```python
from build123d import *

# Parameters (mm, degrees)
ESBO_O1_R                         = 10
RESSALTO_EXTRUS_O1_DEPTH          = 88
ESBO_O1_6_W                       = 24
ESBO_O1_6_H                       = 20
RESSALTO_EXTRUS_O2_DEPTH          = 56
CORTE_EXTRUS_O1_REACH             = 126.957
CORTE_EXTRUS_O1_DIRECTION_2_REACH = 126.957
CORTE_EXTRUS_O2_DEPTH             = 50
CORTE_EXTRUS_O6_REACH             = 126.5
CORTE_EXTRUS_O6_END_RADIUS        = 10
ESBO_O3_R                         = 6
FILETE1_R                         = 3
FILETE2_R                         = 3


with BuildPart() as part:
    # Esboço1 → Ressalto-extrusão1 (new body)
    with BuildSketch(Plane.XY):
        with BuildLine():
            Line((-60, 25), (-48, 25))
            Line((-48, 25), (-48, 35))
            Line((-48, 35), (-42, 35))
            Line((-42, 35), (-42, 50))
            Line((-42, 50), (-18, 50))
            Line((-18, 50), (-18, 35))
            Line((-18, 35), (-12, 35))
            Line((-12, 35), (-12, 25))
            Line((-12, 25), (0, 25))
            ThreePointArc((0, 25), (12.5, 12.5), (0, 0))
            Line((0, 0), (-60, 0))
            ThreePointArc((-60, 0), (-72.5, 12.5), (-60, 25))
        make_face()
        with Locations((-30, 25)):
            Circle(ESBO_O1_R, mode=Mode.SUBTRACT)
    extrude(amount=-RESSALTO_EXTRUS_O1_DEPTH)

    # Esboço1<6> → Ressalto-extrusão2 (add)
    with BuildSketch(Plane.XY):
        with Locations((-30, 60)):
            Rectangle(ESBO_O1_6_W, ESBO_O1_6_H)
    extrude(amount=-RESSALTO_EXTRUS_O2_DEPTH)

    # Esboço2 → Corte-extrusão1 (cut, up to next)
    with BuildSketch(Plane.ZY.offset(42), mode=Mode.PRIVATE) as corte_extrus_o1_sk1:
        Polygon((-40.414518843, 70), (0, 0), (0, 70), align=None)
    corte_extrus_o1_tool1 = extrude(corte_extrus_o1_sk1.sketch, amount=-CORTE_EXTRUS_O1_REACH, mode=Mode.PRIVATE) & part.part
    add(corte_extrus_o1_tool1.solids().sort_by_distance((-42, 46.666667, -13.471506))[0], mode=Mode.SUBTRACT)

    # Esboço2 → Corte-extrusão1 direction 2 (cut, up to next)
    with BuildSketch(Plane.ZY.offset(42), mode=Mode.PRIVATE) as corte_extrus_o1_direction_2_sk1:
        Polygon((-40.414518843, 70), (0, 0), (0, 70), align=None)
    corte_extrus_o1_direction_2_tool1 = extrude(corte_extrus_o1_direction_2_sk1.sketch, amount=CORTE_EXTRUS_O1_DIRECTION_2_REACH, mode=Mode.PRIVATE) & part.part
    add(corte_extrus_o1_direction_2_tool1.solids().sort_by_distance((-42, 46.666667, -13.471506))[0], mode=Mode.SUBTRACT)

    # Esboço1<8> → Corte-extrusão2 (cut)
    with BuildSketch(Plane.XY):
        Polygon((-36, 45), (-24, 45), (-30, 60), align=None)
    extrude(amount=-CORTE_EXTRUS_O2_DEPTH, mode=Mode.SUBTRACT)

    # Corte-extrusão6: up to this cylinder (the profile starts outside it)
    corte_extrus_o6_end = Plane(origin=(-30, 25, -76), z_dir=(0, 0, 1)) * Cylinder(CORTE_EXTRUS_O6_END_RADIUS, 274, mode=Mode.PRIVATE)
    # Esboço3 → Corte-extrusão6 (cut, up to the surface)
    with BuildSketch(Plane(origin=(0, 50, 0), x_dir=(1, 0, 0), z_dir=(0, 1, 0)), mode=Mode.PRIVATE) as corte_extrus_o6_sk1:
        with Locations(Location((-30, 76, 0), (0, 0, 270))):
            Circle(ESBO_O3_R)
    corte_extrus_o6_tool1 = extrude(corte_extrus_o6_sk1.sketch, amount=-CORTE_EXTRUS_O6_REACH, mode=Mode.PRIVATE) - corte_extrus_o6_end
    add(corte_extrus_o6_tool1.solids().sort_by_distance((-30, 50, -76))[0], mode=Mode.SUBTRACT)

    # Filete1
    filete1_edges = [part.edges().sort_by_distance(p)[0] for p in [
        (-30, 70, -56),
    ]]
    fillet(filete1_edges, radius=FILETE1_R)

    # Filete2
    filete2_edges = [part.edges().sort_by_distance(p)[0] for p in [
        (-30, 50, -88),
    ]]
    fillet(filete2_edges, radius=FILETE2_R)


solid = part.part
```
Check sheet for the modelled part. Datum: model origin and axes. Units: mm. A direction names the side the tool comes from. Coordinates: 2 decimals unless noted, no trailing zeros. Write each loop counter-clockwise with the first axis right and the second up, starting at its lowest first coordinate (ties: lowest second). Pieces come first, ordered by that corner, then holes. Notation, with made-up numbers: M 74,34.25 L 119,34.25 A8 cw 119,41.25 Z; hole C -34,54.25 d8. An arc over 180 degrees is marked long. Write item = value, one per line. Start each with the question number.
1. Mould release check, pull along X, two halves, no side actions. Record for faces 1 (the flat face through (-12, 30, -51)), 2 (the flat face through (-32.96, 52.6, -40.49)), 3 (the flat face through (-48, 30, -51)), 4 (the cylindrical face through (-29.83, 69.14, -55.1)): pulls with the +X half, pulls with the -X half, needs draft (parallel to the pull), parting line crosses it, or undercut.
2. Sectioned sample at C-C (z = -76). Record the cut outline in (x, y).
3. Sectioned sample at D-D (x = -56.5). Record the cut outline in (y, z), then the cut area to 3 significant figures.
4. Tool access check on faces 5 (the flat face through (-30, 45, -38)), 6 (the flat face through (-18, 48, -54)), 7 (the flat face through (-30, 59, -56)). Record the directions out of +Z, -Z, +X, -X, +Y, -Y that give a thin tool (end or side, any length) a straight path to the whole face; none if there is none.
5. Sectioned sample at A-A (z = -65.5). Record the cut outline in (x, y).
6. Sectioned sample at B-B (z = -44.5). Record the cut outline in (x, y).
7. Thickness scan on probe 1 along X at (y, z) = (46.25, -76); probe 2 along Y at (x, z) = (-30, -67); probe 3 along Y at (x, z) = (-30, -34). Record the ranges inside material, lowest first.
8. Go/stop test with flat-tipped pins: pin 1 (19 mm diameter, centred on x = -31.5, z = -65, fed in from +Y); pin 2 (8 mm diameter, centred on x = -57, z = -51, fed in from -Y); pin 3 (8.5 mm diameter, centred on x = -33, y = 59.5, fed in from -Z); pin 4 (5 mm diameter, centred on x = -14.5, z = -49, fed in from +Y). Record where each tip stops, or that it passes through.
The answers:
q1.face_1 = pulls with the +X half
q1.face_2 = undercut
q1.face_3 = pulls with the -X half
q1.face_4 = needs draft
q2.outline = M -60,0 L 0,0 A12.5 ccw 0,25 L -12,25 L -12,35 L -18,35 L -18,50 L -24,50 L -24,33 A10 cw long -36,33 L -36,50 L -42,50 L -42,35 L -48,35 L -48,25 L -60,25 A12.5 ccw Z
q3.outline = M 0,-88 L 25,-88 L 25,-14.43 L 0,0 Z
q3.area = 2,020 mm²
q4.face_5 = +Z
q4.face_6 = +Z, -Z, +X, +Y
q4.face_7 = -Z, +X, -X, +Y
q5.outline = M -60,0 L 0,0 A12.5 ccw 0,25 L -12,25 L -12,35 L -18,35 L -18,50 L -42,50 L -42,35 L -48,35 L -48,25 L -60,25 A12.5 ccw Z; hole C -30,25 d20
q6.outline = M -60,0 L 0,0 A12.5 ccw 0,25 L -12,25 L -12,35 L -18,35 L -18,70 L -42,70 L -42,35 L -48,35 L -48,25 L -60,25 A12.5 ccw Z; hole C -30,25 d20; hole M -36,45 L -24,45 L -30,60 Z
q7.probe_1 = -42 to -36, -24 to -18
q7.probe_2 = 0 to 15, 35 to 50
q7.probe_3 = 0 to 15, 35 to 45
q8.pin_1 = 68.66
q8.pin_2 = 0
q8.pin_3 = -56
q8.pin_4 = 35
